```python
from build123d import *

# Parameters (mm, degrees)
F3_DEPTH = 20
F4_SIZE  = 5
F5_R     = 1


with BuildPart() as f3:
    # F2 (on face) → F3 (new body)
    with BuildSketch(Plane.YZ.offset(-138.1125)):
        Polygon((26.8, -39.5), (6.8, -39.5), (6.8, -110.5), (-1, -110.5), (-1, -80.5), (-11, -60.5), (-11, -140.5), (26.8, -140.5), (26.8, -120.5), (26.8, -59.5), align=None)
    extrude(amount=F3_DEPTH)

    # F4
    f4_edges = [f3.edges().sort_by_distance(p)[0] for p in [
        (-128.1125, 26.8, -39.5),
        (-128.1125, 6.8, -39.5),
        (-128.1125, -11, -140.5),
        (-128.1125, 26.8, -140.5),
    ]]
    chamfer(f4_edges, length=F4_SIZE)

    # F5
    f5_edges = [f3.edges().sort_by_distance(p)[0] for p in [
        (-128.1125, -11, -60.5),
        (-128.1125, -1, -80.5),
    ]]
    fillet(f5_edges, radius=F5_R)


solid = f3.part
```
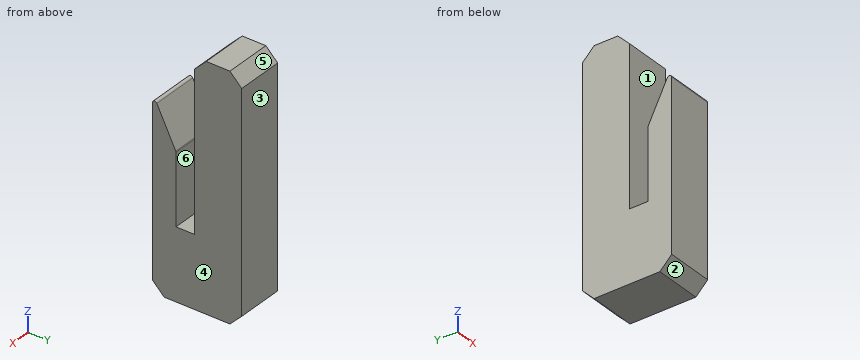
Check sheet for the modelled part. Datum: model origin and axes. Units: mm. Face numbers are marked on the shaded views. A direction names the side the tool comes from. Coordinates: 2 decimals unless noted, no trailing zeros. Write each loop counter-clockwise with the first axis right and the second up, starting at its lowest first coordinate (ties: lowest second). Pieces come first, ordered by that corner, then holes. Notation, with made-up numbers: (52, 12) - (96, 12) arc R16 cw to (96, 26) - close; hole circle Ø5 at (44.5, 69). An arc over 180 degrees is marked (long way). One line per question, with ' | ' between items.
Item 1: Access from +Z, -Z, +X, -X, +Y, -Y to the whole of each face (thin tool, end or side, straight path). Record for the marked faces 5 and 6.
Determined:
face 5: +Z, +X, -X, +Y | face 6: +Z, +X, -X
Item 2: Gauge pin test, flat ends, axial feed: P1, Ø4, axis at x = -124.5, y = 4.5, coming from the +Z side; P2, Ø5, axis at x = -127.5, y = -6.5, coming from the -Z side. Record the tip position at first contact, or that the pin passes through.
Determined:
P1: stops at z = -110.5 | P2: stops at z = -140.5
Item 3: Sectioned sample at A-A on z = -75.5. Record the boundary of the cut face in (x, y), plus the area to 3 significant figures.
Determined:
outline: (-138.11, -11) - (-118.11, -11) - (-118.11, -3.5) - (-138.11, -3.5) - close; (-138.11, 6.8) - (-118.11, 6.8) - (-118.11, 26.8) - (-138.11, 26.8) - close | area: 550 mm2
Item 4: Thickness scan on line 1 (Y direction, x = -134, z = -109.5); line 2 (Y direction, x = -124, z = -70.5); line 3 (Z direction, x = -128, y = 0). Record the ranges inside material, lowest first. Write a range as [from, to].
Determined:
line 1: y = [-11, -1], [6.8, 26.8] | line 2: y = [-11, -6], [6.8, 26.8] | line 3: z = [-140.5, -110.5]
Item 5: Mould release check, pull along Y, two halves, no side actions. Record for the marked faces 1, 2, 3 and 4: pulls with the +Y half, pulls with the -Y half, needs draft (parallel to the pull), parting line crosses it, or undercut.
Determined:
face 1: undercut | face 2: pulls with the -Y half | face 3: pulls with the +Y half | face 4: needs draft
Item 6: Sectioned sample at D-D on y = -3.5. Record the boundary of the cut face in (x, z), plus the area to 3 significant figures.
Determined:
outline: (-138.11, -140.5) - (-118.11, -140.5) - (-118.11, -75.5) - (-138.11, -75.5) - close | area: 1,300 mm2
Item 7: Sectioned sample at C-C on z = -101. Record the boundary of the cut face in (x, y).
Determined:
outline: (-138.11, -11) - (-118.11, -11) - (-118.11, -1) - (-138.11, -1) - close; (-138.11, 6.8) - (-118.11, 6.8) - (-118.11, 26.8) - (-138.11, 26.8) - close
Item 8: Sectioned sample at B-B on x = -130.5. Record the boundary of the cut face in (y, z).
Determined:
outline: (-11, -135.5) - (-6, -140.5) - (21.8, -140.5) - (26.8, -135.5) - (26.8, -44.5) - (21.8, -39.5) - (11.8, -39.5) - (6.8, -44.5) - (6.8, -110.5) - (-1, -110.5) - (-1, -80.74) arc R1 ccw to (-1.11, -80.29) - (-9.11, -64.29) arc R1 ccw to (-11, -64.74) - close
